from build123d import *

# Parameters (mm, degrees)
F7_DEPTH = 5
F0_DEPTH = 18
F2_DEPTH = 15
F5_R     = 3
F8_DEPTH = 25


# Not quite as in the source:
# - a feature names something its author has since deleted; it is built from what else it names


with BuildPart() as f7:
    # F6 (on Top) → F7 (new body)
    with BuildSketch(Plane.XY):
        Polygon((0, -23.2909718978), (7.9219618343, -23.2909718978), (35.9808959381, 59.2037256741), (21.7798681683, 64.0339234217), (0, 0), align=None)
    extrude(amount=F7_DEPTH)

    # F6 (on Top) → F0 (join)
    with BuildSketch(Plane.XY):
        Polygon((21.7798681683, 64.0339234217), (35.9808959381, 59.2037256741), (39.2010277698, 68.6710775207), (25, 73.5012752683), align=None)
    extrude(amount=F0_DEPTH)

    # F1 (on face) → F2 (join, through all)
    with BuildSketch(Plane(origin=(0, 0, 0), x_dir=(-0.3220131832, -0.9467351847, 0), z_dir=(-0.9467351847, 0.3220131832, 0))):
        Polygon((-65.6365729928, 13), (-67.6365729928, 18), (-67.6365729928, 13), align=None)
    extrude(amount=-F2_DEPTH)

    # F3: F7 across face


with BuildPart() as f7_1:
    add(f7.part)
    add(f7.part.mirror(Plane(origin=(0, -11.6454859489, 2.5), x_dir=(0, -1, 0), z_dir=(-1, 0, 0))))

    # F4: F7 across face


with BuildPart() as f7_2:
    add(f7_1.part)
    add(f7_1.part.mirror(Plane(origin=(0, -23.2909718978, 2.5), x_dir=(1, 0, 0), z_dir=(0, -1, 0))))

    # F5 (on face) → F8 (cut)
    with BuildSketch(Plane.XY.offset(5)):
        with Locations((0, -23.2909718978)):
            Circle(F5_R)
    extrude(amount=-F8_DEPTH, mode=Mode.SUBTRACT)


solid = f7_2.part
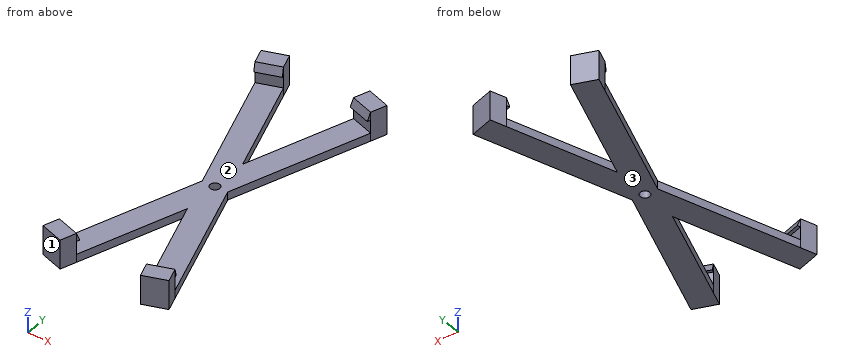
Geometry check sheet. Reference: the model listing, model coordinates, mm. Face numbers are marked on the shaded views. Give positions to 0.01 mm unless a question says otherwise; leave off trailing zeros. Loops run counter-clockwise (first coordinate to the right, second up) from the corner with the lowest first, then second, coordinate; pieces in that order, holes last. Notation, with made-up numbers: (-20.75, 27.25) -> (-3.75, 27.25) arc R16 cw to (-3.75, 33.25) -> close; hole circle Ø3 at (-24, 72.25). An arc over 180 degrees is marked (long way). Answer in a Markdown table with one row per item. Add a question column.
1) Draft check along Y on the marked faces 1, 2 and 3. Enter one of: pulls with the +Y half, pulls with the -Y half, needs draft (parallel to the pull), parting line crosses it, or undercut.
2) Cross-section at C-C on y = 55.5. Record the boundary of the cut face in (x, z), and give its area (3 significant figures).
3) Material ranges on probe 1 along X at (y, z) = (64, 2.75); probe 2 along Y at (x, z) = (28, 5.75); probe 3 along X at (y, z) = (-89, 4.75), recorded low to high. Write a range as from..to.
4) Cross-section at B-B on x = -15.5. Record the boundary of the cut face in (y, z).
5) Gauge pin test, flat ends, axial feed: P1, Ø2, axis at x = -30, y = -107.5, coming from the -Z side; P2, Ø12, axis at x = -13.5, y = -55.5, coming from the +Z side; P3, Ø10, axis at y = -34.5, z = 2, coming from the -X side; P4, Ø5, axis at y = 19.5, z = 9, coming from the -X side. Record the tip position at first contact, or that the pin passes through.
6) Cross-section at A-A on z = 2.5. Record the boundary of the cut face in (x, y), and give its area (3 significant figures).
Outcome:
| question | item | result |
|---|---|---|
| 1 | face 1 | pulls with the -Y half |
| 1 | face 2 | undercut |
| 1 | face 3 | needs draft |
| 2 | outline | (-34.72, 0) -> (-18.88, 0) -> (-18.88, 5) -> (-34.72, 5) -> close; (18.88, 0) -> (34.72, 0) -> (34.72, 5) -> (18.88, 5) -> close |
| 2 | area | 158 mm^2 |
| 3 | probe 1 | x = -37.61..-21.77, 21.77..37.61 |
| 3 | probe 2 | y = -119.06..-108.5, 61.92..72.48 |
| 3 | probe 3 | x = -30.27..-14.43, 14.43..30.27 |
| 4 | outline | (-92.15, 0) -> (-45.57, 0) -> (-45.57, 5) -> (-92.15, 5) -> close; (-1.01, 0) -> (45.57, 0) -> (45.57, 5) -> (-1.01, 5) -> close |
| 5 | P1 | stops at z = 0 |
| 5 | P2 | stops at z = 5 |
| 5 | P3 | stops at x = -13.44 |
| 5 | P4 | passes through |
| 6 | outline | (-39.2, -115.25) -> (-25, -120.08) -> (0, -46.58) -> (25, -120.08) -> (39.2, -115.25) -> (7.92, -23.29) -> (39.2, 68.67) -> (25, 73.5) -> (0, 0) -> (-25, 73.5) -> (-39.2, 68.67) -> (-7.92, -23.29) -> close; hole circle Ø6 at (0, -23.29) |
| 6 | area | 5,580 mm^2 |
